The listing builds one solid part. Answer for the finished solid, in the listing's coordinates (mm). Coordinates: 2 decimals unless noted, no trailing zeros. Write each loop counter-clockwise with the first axis right and the second up, starting at its lowest first coordinate (ties: lowest second). Pieces come first, ordered by that corner, then holes.
(1) Straight lines are drawn through the part: line 1 (Y direction, x = -130, z = 1.65); line 2 (Y direction, x = 70, z = 1.45); line 3 (X direction, y = -37.5, z = 1.5). For each, find the intervals that lie inside material, in ascending order.
(2) The part is cut by section A-A on x = -93.5. Determine the outline of the cut face in (y, z), plus the area to 3 significant figures.
(3) Given P1, Ø0.9, axis at x = 81.5, z = 1.5, coming from the -Y side; P2, Ø0.9, axis at x = 78, z = 1, coming from the +Y side; P3, Ø1.5, axis at y = 47, z = 2, coming from the +X side, each flat-ended and moving along its own axis, determine where each tip first touches the part or whether it passes through.
(4) The part is cut by section B-B on z = 1.9. Give the number of separate pieces and of enclosed holes in the cut face, plus the area to 4 significant figures.
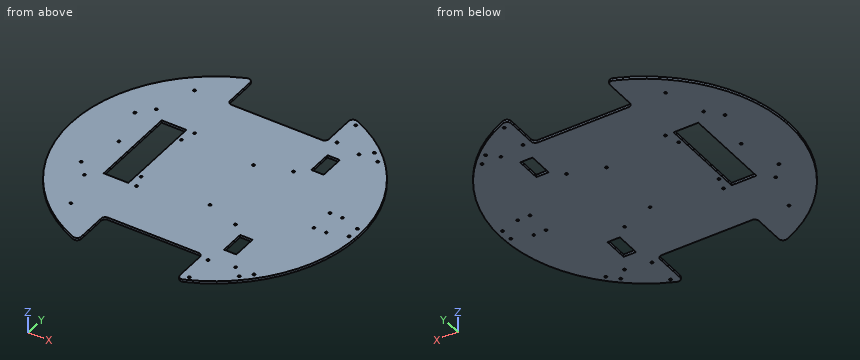
from build123d import *

# Parameters (mm, degrees)
SKETCH_1_R           = 175
EXTRUDE_1_DEPTH      = 3
CUT_EXTRUDE_1_DEPTH  = 3
FILLET_1_R           = 5
FILLET_2_R           = 5
FILLET_3_R           = 5
SKETCH_5_R           = 1.5
CUT_EXTRUDE_4_DEPTH  = 3
SKETCH_6_R           = 1.5
CUT_EXTRUDE_5_DEPTH  = 3
SKETCH_7_W           = 30
SKETCH_7_H           = 108
CUT_EXTRUDE_6_DEPTH  = 3
SKETCH_8_R           = 1.5
CUT_EXTRUDE_7_DEPTH  = 3
SKETCH_9_R           = 1.5
CUT_EXTRUDE_8_DEPTH  = 10
SKETCH_10_R          = 1.6
CUT_EXTRUDE_9_DEPTH  = 10
SKETCH_11_W          = 15
SKETCH_11_H          = 30
CUT_EXTRUDE_10_DEPTH = 10
SKETCH_13_R          = 1.5
CUT_EXTRUDE_12_DEPTH = 4
SKETCH_14_R          = 1.6
CUT_EXTRUDE_14_DEPTH = 4


with BuildPart() as part:
    # ｽｹｯﾁ1 → ﾎﾞｽ - 押し出し1 (new body)
    with BuildSketch(Plane.XY):
        Circle(SKETCH_1_R)
    extrude(amount=EXTRUDE_1_DEPTH)

    # ｽｹｯﾁ2 → ｶｯﾄ - 押し出し1 (cut)
    with BuildSketch(Plane.XY.offset(3)):
        with BuildLine():
            Line((-60, 115), (0, 115))
            Line((0, 115), (0, 175))
            ThreePointArc((0, 175), (-30.465194158, 172.327803749), (-60, 164.392822228))
            Line((-60, 164.392822228), (-60, 115))
        make_face()
        with BuildLine():
            Line((0, 175), (0, 115))
            Line((0, 115), (60, 115))
            Line((60, 115), (60, 164.392822228))
            ThreePointArc((60, 164.392822228), (30.465194158, 172.327803749), (0, 175))
        make_face()
        with BuildLine():
            Line((0, -175), (0, -115))
            Line((0, -115), (-60, -115))
            Line((-60, -115), (-60, -164.392822228))
            ThreePointArc((-60, -164.392822228), (-30.465194158, -172.327803749), (0, -175))
        make_face()
        with BuildLine():
            Line((60, -115), (0, -115))
            Line((0, -115), (0, -175))
            ThreePointArc((0, -175), (30.465194158, -172.327803749), (60, -164.392822228))
            Line((60, -164.392822228), (60, -115))
        make_face()
    extrude(amount=-CUT_EXTRUDE_1_DEPTH, mode=Mode.SUBTRACT)

    # ﾌｨﾚｯﾄ1
    fillet_1_edges = [part.edges().sort_by_distance(p)[0] for p in [
        (-60, 164.392822228, 1.5),
    ]]
    fillet(fillet_1_edges, radius=FILLET_1_R)

    # ﾌｨﾚｯﾄ2
    fillet_2_edges = [part.edges().sort_by_distance(p)[0] for p in [
        (-60, 115, 1.5),
        (60, 164.392822228, 1.5),
        (60, 115, 1.5),
    ]]
    fillet(fillet_2_edges, radius=FILLET_2_R)

    # ﾌｨﾚｯﾄ3
    fillet_3_edges = [part.edges().sort_by_distance(p)[0] for p in [
        (-60, -115, 1.5),
        (60, -115, 1.5),
        (60, -164.392822228, 1.5),
        (-60, -164.392822228, 1.5),
    ]]
    fillet(fillet_3_edges, radius=FILLET_3_R)

    # ｽｹｯﾁ5 → ｶｯﾄ - 押し出し4 (cut)
    with BuildSketch(Plane.XY.offset(3)):
        with Locations((-100, -115)):
            Circle(SKETCH_5_R)
        with Locations((100, -115)):
            Circle(SKETCH_5_R)
        with Locations((100, 115)):
            Circle(SKETCH_5_R)
        with Locations((-100, 115)):
            Circle(SKETCH_5_R)
    extrude(amount=-CUT_EXTRUDE_4_DEPTH, mode=Mode.SUBTRACT)

    # ｽｹｯﾁ6 → ｶｯﾄ - 押し出し5 (cut)
    with BuildSketch(Plane.XY.offset(3)):
        with Locations((-60, 54)):
            Circle(SKETCH_6_R)
        with Locations((60, 54)):
            Circle(SKETCH_6_R)
        with Locations((-60, -54)):
            Circle(SKETCH_6_R)
        with Locations((60, -54)):
            Circle(SKETCH_6_R)
    extrude(amount=-CUT_EXTRUDE_5_DEPTH, mode=Mode.SUBTRACT)

    # ｽｹｯﾁ7 → ｶｯﾄ - 押し出し6 (cut)
    with BuildSketch(Plane.XY.offset(3)):
        with Locations((-85, 0)):
            Rectangle(SKETCH_7_W, SKETCH_7_H)
    extrude(amount=-CUT_EXTRUDE_6_DEPTH, mode=Mode.SUBTRACT)

    # ｽｹｯﾁ8 → ｶｯﾄ - 押し出し7 (cut)
    with BuildSketch(Plane.XY.offset(3)):
        with Locations((-115, -67)):
            Circle(SKETCH_8_R)
        with Locations((-116.822468618, 0)):
            Circle(SKETCH_8_R)
        with Locations((-115, 67)):
            Circle(SKETCH_8_R)
    extrude(amount=-CUT_EXTRUDE_7_DEPTH, mode=Mode.SUBTRACT)

    # ｽｹｯﾁ9 → ｶｯﾄ - 押し出し8 (cut)
    with BuildSketch(Plane.XY.offset(3)):
        with Locations((-65, 37)):
            Circle(SKETCH_9_R)
        with Locations((20, 41)):
            Circle(SKETCH_9_R)
        with Locations((-65, -38)):
            Circle(SKETCH_9_R)
        with Locations((20, -40)):
            Circle(SKETCH_9_R)
    extrude(amount=-CUT_EXTRUDE_8_DEPTH, mode=Mode.SUBTRACT)

    # ｽｹｯﾁ10 → ｶｯﾄ - 押し出し9 (cut)
    with BuildSketch(Plane.XY.offset(3)):
        with Locations((111.643659725, -125.921059639)):
            Circle(SKETCH_10_R)
        with Locations((122.679794489, -115.037952538)):
            Circle(SKETCH_10_R)
        with Locations((168, 7.75)):
            Circle(SKETCH_10_R)
        with Locations((168, -7.75)):
            Circle(SKETCH_10_R)
        with Locations((111.56768007, 125.844011632)):
            Circle(SKETCH_10_R)
        with Locations((122.679794489, 115.037952538)):
            Circle(SKETCH_10_R)
    extrude(amount=-CUT_EXTRUDE_9_DEPTH, mode=Mode.SUBTRACT)

    # ｽｹｯﾁ11 → ｶｯﾄ - 押し出し10 (cut)
    with BuildSketch(Plane.XY.offset(3)):
        with Locations((81.317279836, 81.317279836)):
            Rectangle(SKETCH_11_W, SKETCH_11_H)
        with Locations((81.317279836, -81.317279836)):
            Rectangle(SKETCH_11_W, SKETCH_11_H)
    extrude(amount=-CUT_EXTRUDE_10_DEPTH, mode=Mode.SUBTRACT)

    # ｽｹｯﾁ13 → ｶｯﾄ - 押し出し12 (cut, through all)
    with BuildSketch(Plane.XY.offset(3)):
        with Locations((130, 15)):
            Circle(SKETCH_13_R)
        with Locations((145, 15)):
            Circle(SKETCH_13_R)
        with Locations((130, -15)):
            Circle(SKETCH_13_R)
        with Locations((145, -15)):
            Circle(SKETCH_13_R)
    extrude(amount=-CUT_EXTRUDE_12_DEPTH, mode=Mode.SUBTRACT)

    # ｽｹｯﾁ14 → ｶｯﾄ - 押し出し14 (cut, through all)
    with BuildSketch(Plane.XY.offset(3)):
        with Locations((70, 119.792059696)):
            Circle(SKETCH_14_R)
        with Locations((70, 154.792059696)):
            Circle(SKETCH_14_R)
        with Locations((70, -120)):
            Circle(SKETCH_14_R)
        with Locations((70, -155)):
            Circle(SKETCH_14_R)
        with Locations((-130, 50.05)):
            Circle(SKETCH_14_R)
        with Locations((-130, -50.05)):
            Circle(SKETCH_14_R)
    extrude(amount=-CUT_EXTRUDE_14_DEPTH, mode=Mode.SUBTRACT)


solid = part.part
Model answer:
1. line 1: y = -117.15 to -51.65, -48.45 to 48.45, 51.65 to 117.15
1. line 2: y = -160.39 to -156.6, -153.4 to -121.6, -118.4 to 118.19, 121.39 to 153.19, 156.39 to 160.39
1. line 3: x = -170.93 to -100, -70 to -66.41, -63.59 to 170.93
2. outline: (-147.93, 0) - (-54, 0) - (-54, 3) - (-147.93, 3) - close; (54, 0) - (147.93, 0) - (147.93, 3) - (54, 3) - close
2. area: 564 mm2
3. P1: stops at y = -155.1
3. P2: stops at y = 156.88
3. P3: stops at x = 168.78
4. separate pieces: 1
4. enclosed holes: 34
4. area: 78,250 mm2
